from build123d import *


with BuildPart() as f2:
    # F2: sweep along a path in F1
    with BuildLine(Plane.XY) as f2_path:
        Line((0, 0), (0, 17.78))
    # F0 (on Front) → F2 (sweep)
    with BuildSketch(Plane.XZ):
        Polygon((12.330452, 0.207421), (5.985594, 10.782195), (-6.344858, 10.574774), (-12.330452, -0.207421), (-5.985594, -10.782195), (6.344858, -10.574774), align=None)
    sweep(path=f2_path.line)


solid = f2.part
Here's how the part is built. I have some questions about the finished solid (model axes, mm). Give positions to 0.01 mm unless a question says otherwise; leave off trailing zeros. Order: outer loops, then holes, each group sorted by start corner. A loop starts at its lowest first (then second) coordinate and runs counter-clockwise, first axis right, second up. Notation, with made-up numbers: (41, 86) -> (98, 86) arc R31 ccw to (98, 122) -> close; hole circle Ø6 at (62, -11). An arc over 180 degrees is marked (long way). Use a Markdown table: item, result. Add a question column.
Item 1: Imagine slicing it at C-C on x = 8.5. Please give me the cut outline in (y, z), plus the area to 3 significant figures.
Item 2: Will these pins go through, and if not, where does the flat tip stop? pin 1 (1.5 mm diameter, centred on x = 9.5, y = 16, fed in from -Z); pin 2 (2 mm diameter, centred on y = 9, z = 6.5, fed in from +X); pin 3 (10 mm diameter, centred on x = 5.5, y = 8, fed in from +Z); pin 4 (4 mm diameter, centred on y = 5, z = 4, fed in from -X).
Item 3: I need wall thicknesses on line 1 (X direction, y = 2.5, z = -6.5); line 2 (Z direction, x = -7, y = 8.5); line 3 (Z direction, x = 11, y = 5.5). Which ranges of each line are inside material? Lowest first, please.
Item 4: Imagine slicing it at A-A on y = 7.75. Please give me the cut outline in (x, z), plus the area to 3 significant figures.
Item 5: Imagine slicing it at B-B on z = 6. Please give me the cut outline in (x, y).
Data:
| question | item | result |
|---|---|---|
| 1 | outline | (0, -6.69) -> (17.78, -6.69) -> (17.78, 6.59) -> (0, 6.59) -> close |
| 1 | area | 236 mm² |
| 2 | pin 1 | stops at z = -6.24 |
| 2 | pin 2 | stops at x = 9.15 |
| 2 | pin 3 | stops at z = 10.78 |
| 2 | pin 4 | stops at x = -11.11 |
| 3 | line 1 | x = -8.55 to 8.61 |
| 3 | line 2 | z = -9.09 to 9.39 |
| 3 | line 3 | z = -2.19 to 2.42 |
| 4 | outline | (-12.33, -0.21) -> (-5.99, -10.78) -> (6.34, -10.57) -> (12.33, 0.21) -> (5.99, 10.78) -> (-6.34, 10.57) -> close |
| 4 | area | 395 mm² |
| 5 | outline | (-8.88, 0) -> (8.85, 0) -> (8.85, 17.78) -> (-8.88, 17.78) -> close |
